from build123d import *

# Parameters (mm, degrees)
CYLINDER011_R     = 1.4
CYLINDER011_DEPTH = 14
CYLINDER010_R     = 1.4
CYLINDER010_DEPTH = 14
CYLINDER009_R     = 1.4
CYLINDER009_DEPTH = 14
CYLINDER004_R     = 2
CYLINDER004_DEPTH = 40
CYLINDER005_R     = 2
CYLINDER005_DEPTH = 40
CYLINDER006_R     = 2
CYLINDER006_DEPTH = 40
CYLINDER007_R     = 2
CYLINDER007_DEPTH = 40
CYLINDER_R        = 2
CYLINDER_DEPTH    = 10
BOX004_W          = 2
BOX004_H          = 15
BOX004_DEPTH      = 4
FILLET002_R       = 1.9
BOX003_W          = 2
BOX003_H          = 15
BOX003_DEPTH      = 4
FILLET003_R       = 1.9
CYLINDER008_R     = 1.4
CYLINDER008_DEPTH = 14
BOX005_W          = 5
BOX005_H          = 5
BOX005_DEPTH      = 12
BOX006_W          = 5
BOX006_H          = 5
BOX006_DEPTH      = 12
BOX008_W          = 5
BOX008_H          = 5
BOX008_DEPTH      = 12
CYLINDER012_R     = 2
CYLINDER012_DEPTH = 10
BOX007_W          = 5
BOX007_H          = 12
BOX007_DEPTH      = 12
BOX_W             = 73
BOX_H             = 56
BOX_DEPTH         = 40
FILLET_R          = 4
BOX001_W          = 77
BOX001_H          = 60
BOX001_DEPTH      = 42
FILLET001_R       = 6
CHAMFER_SIZE      = 1
FILLET004_R       = 0.5


with BuildPart() as obj1:
    # Cylinder011 → Cylinder011 (new body)
    with BuildSketch(Plane(origin=(-28, -4.2, 0), x_dir=(1, 0, 0), z_dir=(0, 0, 1))):
        Circle(CYLINDER011_R)
    extrude(amount=CYLINDER011_DEPTH)


with BuildPart() as obj2:
    # Cylinder010 → Cylinder010 (new body)
    with BuildSketch(Plane(origin=(15.6, 8.4, 0), x_dir=(1, 0, 0), z_dir=(0, 0, 1))):
        Circle(CYLINDER010_R)
    extrude(amount=CYLINDER010_DEPTH)


with BuildPart() as obj3:
    # Cylinder009 → Cylinder009 (new body)
    with BuildSketch(Plane(origin=(15.6, -19, 0), x_dir=(1, 0, 0), z_dir=(0, 0, 1))):
        Circle(CYLINDER009_R)
    extrude(amount=CYLINDER009_DEPTH)


with BuildPart() as zylinder:
    # Cylinder004 → Cylinder004 (new body)
    with BuildSketch(Plane(origin=(32, 24, 0), x_dir=(1, 0, 0), z_dir=(0, 0, 1))):
        Circle(CYLINDER004_R)
    extrude(amount=CYLINDER004_DEPTH)


with BuildPart() as zylinder001:
    # Cylinder005 → Cylinder005 (new body)
    with BuildSketch(Plane(origin=(32, -24, 0), x_dir=(1, 0, 0), z_dir=(0, 0, 1))):
        Circle(CYLINDER005_R)
    extrude(amount=CYLINDER005_DEPTH)


with BuildPart() as zylinder002:
    # Cylinder006 → Cylinder006 (new body)
    with BuildSketch(Plane(origin=(-33, 24, 0), x_dir=(1, 0, 0), z_dir=(0, 0, 1))):
        Circle(CYLINDER006_R)
    extrude(amount=CYLINDER006_DEPTH)


with BuildPart() as zylinder003:
    # Cylinder007 → Cylinder007 (new body)
    with BuildSketch(Plane(origin=(-33, -24, 0), x_dir=(1, 0, 0), z_dir=(0, 0, 1))):
        Circle(CYLINDER007_R)
    extrude(amount=CYLINDER007_DEPTH)


with BuildPart() as zylinder004:
    # Cylinder → Cylinder (new body)
    with BuildSketch(Plane(origin=(32, 14, 4), x_dir=(0, 0, -1), z_dir=(1, 0, 0))):
        Circle(CYLINDER_R)
    extrude(amount=CYLINDER_DEPTH)


with BuildPart() as fillet002:
    # Box004 → Box004 (new body)
    with BuildSketch(Plane(origin=(-39, 1, 2), x_dir=(1, 0, 0), z_dir=(0, 0, 1))):
        with Locations((1, 7.5)):
            Rectangle(BOX004_W, BOX004_H)
    extrude(amount=BOX004_DEPTH)

    # Fillet002
    fillet002_edges = [fillet002.edges().sort_by_distance(p)[0] for p in [
        (-38, 1, 2),
        (-38, 1, 6),
        (-38, 16, 2),
        (-38, 16, 6),
    ]]
    fillet(fillet002_edges, radius=FILLET002_R)


with BuildPart() as fillet003:
    # Box003 → Box003 (new body)
    with BuildSketch(Plane(origin=(36, -17, 2), x_dir=(1, 0, 0), z_dir=(0, 0, 1))):
        with Locations((1, 7.5)):
            Rectangle(BOX003_W, BOX003_H)
    extrude(amount=BOX003_DEPTH)

    # Fillet003
    fillet003_edges = [fillet003.edges().sort_by_distance(p)[0] for p in [
        (37, -17, 2),
        (37, -17, 6),
        (37, -2, 2),
        (37, -2, 6),
    ]]
    fillet(fillet003_edges, radius=FILLET003_R)


with BuildPart() as fusion:
    # Cylinder008 → Cylinder008 (new body)
    with BuildSketch(Plane(origin=(-28, -19, 0), x_dir=(1, 0, 0), z_dir=(0, 0, 1))):
        Circle(CYLINDER008_R)
    extrude(amount=CYLINDER008_DEPTH)

    # Fusion: union obj1, obj2, obj3, Zylinder, Zylinder001, Zylinder002, Zylinder003, Zylinder004, Fillet002, Fillet003
    add(obj1.part)
    add(obj2.part)
    add(obj3.part)
    add(zylinder.part)
    add(zylinder001.part)
    add(zylinder002.part)
    add(zylinder003.part)
    add(zylinder004.part)
    add(fillet002.part)
    add(fillet003.part)


with BuildPart() as obj4:
    # Box005 → Box005 (new body)
    with BuildSketch(Plane(origin=(-30.5, -21.5, 0), x_dir=(1, 0, 0), z_dir=(0, 0, 1))):
        with Locations((2.5, 2.5)):
            Rectangle(BOX005_W, BOX005_H)
    extrude(amount=BOX005_DEPTH)


with BuildPart() as obj5:
    # Box006 → Box006 (new body)
    with BuildSketch(Plane(origin=(13.1, -21.5, 0), x_dir=(1, 0, 0), z_dir=(0, 0, 1))):
        with Locations((2.5, 2.5)):
            Rectangle(BOX006_W, BOX006_H)
    extrude(amount=BOX006_DEPTH)


with BuildPart() as obj6:
    # Box008 → Box008 (new body)
    with BuildSketch(Plane(origin=(-30.5, -6.6, 0), x_dir=(1, 0, 0), z_dir=(0, 0, 1))):
        with Locations((2.5, 2.5)):
            Rectangle(BOX008_W, BOX008_H)
    extrude(amount=BOX008_DEPTH)


with BuildPart() as zylinder005:
    # Cylinder012 → Cylinder012 (new body)
    with BuildSketch(Plane(origin=(11, 3, 4), x_dir=(0, 0, -1), z_dir=(1, 0, 0))):
        Circle(CYLINDER012_R)
    extrude(amount=CYLINDER012_DEPTH)


with BuildPart() as cut001:
    # Box007 → Box007 (new body)
    with BuildSketch(Plane(origin=(13.1, -1.1, 0), x_dir=(1, 0, 0), z_dir=(0, 0, 1))):
        with Locations((2.5, 6)):
            Rectangle(BOX007_W, BOX007_H)
    extrude(amount=BOX007_DEPTH)

    # Cut001: cut Zylinder005
    add(zylinder005.part, mode=Mode.SUBTRACT)


with BuildPart() as obj7:
    # Box → Box (new body)
    with BuildSketch(Plane(origin=(-37, -28, 2), x_dir=(1, 0, 0), z_dir=(0, 0, 1))):
        with Locations((36.5, 28)):
            Rectangle(BOX_W, BOX_H)
    extrude(amount=BOX_DEPTH)

    # Fillet
    fillet_edges = [obj7.edges().sort_by_distance(p)[0] for p in [
        (-37, -28, 22),
        (-37, 28, 22),
        (36, -28, 22),
        (36, 28, 22),
    ]]
    fillet(fillet_edges, radius=FILLET_R)


with BuildPart() as obj8:
    # Box001 → Box001 (new body)
    with BuildSketch(Plane(origin=(-39, -30, 0), x_dir=(1, 0, 0), z_dir=(0, 0, 1))):
        with Locations((38.5, 30)):
            Rectangle(BOX001_W, BOX001_H)
    extrude(amount=BOX001_DEPTH)

    # Fillet001
    fillet001_edges = [obj8.edges().sort_by_distance(p)[0] for p in [
        (-39, -30, 21),
        (-39, 30, 21),
        (38, -30, 21),
        (38, 30, 21),
    ]]
    fillet(fillet001_edges, radius=FILLET001_R)

    # Cut: cut obj7
    add(obj7.part, mode=Mode.SUBTRACT)

    # Fusion001: union obj4, obj5, obj6, Cut001
    add(obj4.part)
    add(obj5.part)
    add(obj6.part)
    add(cut001.part)

    # Cut002: cut Fusion
    add(fusion.part, mode=Mode.SUBTRACT)

    # Chamfer
    chamfer_edges = [obj8.edges().sort_by_distance(p)[0] for p in [
        (30, 24, 2),
        (-35, 24, 2),
        (-35, -24, 2),
        (30, -24, 2),
    ]]
    chamfer(chamfer_edges, length=CHAMFER_SIZE)

    # Fillet004
    fillet004_edges = [obj8.edges().sort_by_distance(p)[0] for p in [
        (-39, 0, 42),
        (-37.242641, -28.242641, 42),
        (-37.242641, 28.242641, 42),
        (-0.5, -30, 42),
        (-0.5, 30, 42),
        (36.242641, -28.242641, 42),
        (36.242641, 28.242641, 42),
        (38, 0, 42),
        (-37, 0, 42),
        (-35.828427, -26.828427, 42),
        (-0.5, -28, 42),
        (34.828427, -26.828427, 42),
        (-35.828427, 26.828427, 42),
        (36, 0, 42),
        (-0.5, 28, 42),
        (34.828427, 26.828427, 42),
    ]]
    fillet(fillet004_edges, radius=FILLET004_R)


solid = obj8.part
Can you work these out from the model? Positions are in its coordinate system, mm. A direction names the side the tool comes from. Coordinates: 2 decimals unless noted, no trailing zeros. Loops run counter-clockwise (first coordinate to the right, second up) from the corner with the lowest first, then second, coordinate; pieces in that order, holes last. Notation, with made-up numbers: M 69,24 L 112,24 A11 cw 112,43 Z; hole C 4,0.25 d8. An arc over 180 degrees is marked long. Return JSON: item names as keys, results as strings. Group by question number.
Item 1: I'm going to push flat-ended pins straight in: pin 1 Ø3 at (x, y) = (-11.5, 20) entering from +Z; pin 2 Ø6.5 at (x, y) = (-33, -24) entering from -Z; pin 3 Ø1.5 at (x, y) = (-29, -3) entering from +Z. Where does each tip first touch, or does it pass through?
Item 2: Imagine slicing it at D-D (z = 24). Please give me the cut outline in (x, y), and give its area (3 significant figures).
Item 3: On a 3-axis mill with a long thin cutter (end or side, diameter ignored), from which of +Z, -Z, +X, -X, +Y, -Y can I reach the whole of each face in a straight line? I mean faces 5 (the cylindrical face through (37.014, -2.542, 2.571)), 6 (the flat face through (13.1, 5, 7)), 7 (the cylindrical face through (-37.289, -28.196, 21.04)). Say none if no direction works.
Item 4: Imagine slicing it at B-B (x = -28). Please give me the cut outline in (y, z), and give its area (3 significant figures).
Item 5: Imagine slicing it at A-A (x = 15.6). Give the number of separate pieces and of enclosed holes in the cut face, and give its area (3 significant figures).
Item 6: If I drill on L1, parallel to X at y = -19, z = 9; L2, parallel to Y at x = -28, z = 9.25; L3, parallel to Y at x = 14, z = 4, over which ranges is the centre line in solid material (lowest first)? Write a range as from..to.
Item 7: Thinking about a two-plate mould opening in X: for faces 1 (the cylindrical face through (-37.289, 28.196, 21.04)), 2 (the flat face through (13.1, -19, 7)), 3 (the flat face through (-38, 9, 6)), 4 (the cylindrical face through (33.908, -23.399, 0.493)), which applies, released by +X, released by -X, zero draft, split by the parting line, or undercut?
Verdict:
{
 "1": {"pin 1": "stops at z = 2", "pin 2": "stops at z = 0", "pin 3": "stops at z = 12"},
 "2": {"outline": "M -39,-24 A6 ccw -33,-30 L 32,-30 A6 ccw 38,-24 L 38,24 A6 ccw 32,30 L -33,30 A6 ccw -39,24 Z; hole M -37,-24 A4 ccw -33,-28 L 32,-28 A4 ccw 36,-24 L 36,24 A4 ccw 32,28 L -33,28 A4 ccw -37,24 Z", "area": "515 mm^2"},
 "3": {"face 5": "+X", "face 6": "+Z", "face 7": "+Z, -Z, -X, -Y"},
 "4": {"outline": "M -30,0 L -20.4,0 L -20.4,12 L -21.5,12 L -21.5,2 L -28,2 L -28,41.5 A0.5 ccw -28.5,42 L -29.5,42 A0.5 ccw -30,41.5 Z; M -17.6,0 L -5.6,0 L -5.6,12 L -6.6,12 L -6.6,2 L -16.5,2 L -16.5,12 L -17.6,12 Z; M -2.8,0 L 30,0 L 30,41.5 A0.5 ccw 29.5,42 L 28.5,42 A0.5 ccw 28,41.5 L 28,2 L -1.6,2 L -1.6,12 L -2.8,12 Z", "area": "313 mm^2"},
 "5": {"separate pieces": "3", "enclosed holes": "1", "area": "370 mm^2"},
 "6": {"L1": "x = -39..-37, -30.5..-29.4, -26.6..-25.5, 13.1..14.2, 17..18.1, 36..38", "L2": "y = -30..-28, -21.5..-20.4, -17.6..-16.5, -6.6..-5.6, -2.8..-1.6, 28..30", "L3": "y = -30..-28, -21.5..-16.5, -1.1..1, 5..10.9, 28..30"},
 "7": {"face 1": "released by -X", "face 2": "undercut", "face 3": "zero draft", "face 4": "undercut"}
}
